Geometry: final body of the model. Coordinates: model frame, mm. A direction names the side the tool comes from. Round coordinates to 2 decimals unless told otherwise and drop trailing zeros. Loops run counter-clockwise (first coordinate to the right, second up) from the corner with the lowest first, then second, coordinate; pieces in that order, holes last. Notation, with made-up numbers: M 25,50.5 L 35,50.5 A24 ccw 35,74.5 Z; hole C 79.25,67 d8. An arc over 180 degrees is marked long. Write each question's results on one line, items separated by ' | '.
```python
from build123d import *

# Parameters (mm, degrees)
FILLET1_R          = 6
SKETCH2_W          = 7.935978024
SKETCH2_H          = 33.147969744
CUT_EXTRUDE1_DEPTH = 20
SKETCH3_R          = 4
CUT_EXTRUDE2_DEPTH = 108.70389036


with BuildPart() as part:
    # Sketch1 → Revolve1 (revolve)
    with BuildSketch(Plane.XY, mode=Mode.PRIVATE) as revolve1_sk:
        Polygon((0, 0), (11.5, 0), (11.5, 28), (22.5, 28), (22.5, 31), (5, 31), (5, 101), (0, 101), align=None)
    revolve(revolve1_sk.sketch.rotate(Axis((0, 101, 0), (0, -1, 0)), 180), axis=Axis((0, 101, 0), (0, -1, 0)))

    # Fillet1
    fillet1_edges = [part.edges().sort_by_distance(p)[0] for p in [
        (11.5, 0, 0),
    ]]
    fillet(fillet1_edges, radius=FILLET1_R)

    # Sketch2 → Cut-Extrude1 (cut)
    with BuildSketch(Plane.XZ):
        Polygon((15.765034156, 15.943007174), (14.41031705, -17.177268183), (6.480969359, -16.852934437), (7.835686465, 16.26734092), align=None)
        with Locations((-11.132302547, 0)):
            Rectangle(SKETCH2_W, SKETCH2_H)
    extrude(amount=-CUT_EXTRUDE1_DEPTH, mode=Mode.SUBTRACT)

    # Sketch3 → Cut-Extrude2 (cut, through all)
    with BuildSketch(Plane(origin=(7.158327912, 0, -0.292796759), x_dir=(-0.040868780695827604, 0, -0.9991645223707837), z_dir=(0.9991645223707837, 0, -0.040868780695827604))):
        with Locations((0, 10)):
            Circle(SKETCH3_R)
    extrude(amount=-CUT_EXTRUDE2_DEPTH, mode=Mode.SUBTRACT)


solid = part.part
```
1. Pin query (flat end, axial travel): P1, Ø6, axis at x = 3.5, z = -17, coming from the +Y side; P2, Ø20, axis at y = 5.5, z = 0, coming from the -X side; P3, Ø5, axis at x = -10, z = -1.5, coming from the -Y side. Return the tip coordinate at first contact, or that it passes through.
Answer key:
P1: stops at y = 31 | P2: stops at x = -7.16 | P3: stops at y = 20
2. Ray query, probe 1 along Y at (x, z) = (-17.5, 2); probe 2 along X at (y, z) = (13.5, 4.5); probe 3 along Z at (x, y) = (10.5, 26). Return the intervals inside material, ascending.
Answer key:
probe 1: y = 28 to 31 | probe 2: x = -7.16 to 7.35 | probe 3: z = -4.69 to 4.69
3. Draft query along Y for faces 1 (the face through (0.03, 13.966, 0.52)), 2 (the face through (10, 28, 10)), 3 (the face through (0.3, 31, -5.3)), 4 (the face through (5, 66, 0)). Return one class per face: pulls with the +Y half, pulls with the -Y half, needs draft (parallel to the pull), parting line crosses it, or undercut.
Answer key:
face 1: undercut | face 2: pulls with the -Y half | face 3: pulls with the +Y half | face 4: needs draft
4. Section D-D (z = -17.5). Output: boundary loops of the cut face in (x, y), then the cut area to 3 significant figures.
Answer key:
outline: M -14.14,28 L 14.14,28 L 14.14,31 L -14.14,31 Z | area: 84.9 mm²
5. Access query for faces 5 (the face through (0, 0, 0)), 6 (the face through (-9, 20, 0)), 7 (the face through (7.153, 14.371, -0.419)), 8 (the face through (-10.97, 22.04, -3.45)). Directions: +Z, -Z, +X, -X, +Y, -Y. A direction counts if a zero-diameter tool reaches every point of the face in a straight line with its end or side. Return the directions, or none.
Answer key:
face 5: +Z, -Z, +X, -X, -Y | face 6: +Z, -Z, -X, -Y | face 7: -Z, +X, -Y | face 8: -Y
6. Section A-A (y = 8.5). Output: boundary loops of the cut face in (x, z), then the cut area to 3 significant figures.
Answer key:
outline: M -7.16,-9 A11.5 ccw 6.79,-9.28 L 7.01,-4 L -7.16,-3.42 Z; M -7.16,4 L 7.31,3.41 L 7.53,8.7 A11.5 ccw -7.16,9 Z | area: 200 mm²
7. Section C-C (y = 59). Output: boundary loops of the cut face in (x, z), then the cut area to 3 significant figures.
Answer key:
outline: C 0,0 d10 | area: 78.5 mm²
8. Section B-B (x = -10.5). Output: boundary loops of the cut face in (y, z), then the cut area to 3 significant figures.
Answer key:
outline: M 20,-4.69 L 28,-4.69 L 28,-19.9 L 31,-19.9 L 31,19.9 L 28,19.9 L 28,4.69 L 20,4.69 Z | area: 194 mm²
